Design review of the part built by this model. Coordinates are the model's own, in mm. Face numbers are marked on the shaded views. A direction names the side the tool comes from. Give positions to 0.01 mm unless a question says otherwise; leave off trailing zeros. Write each loop counter-clockwise with the first axis right and the second up, starting at its lowest first coordinate (ties: lowest second). Pieces come first, ordered by that corner, then holes. Notation, with made-up numbers: (50, 27.5) -> (105, 27.5) arc R14 ccw to (105, 33.5) -> close; hole circle Ø11 at (17, -11.5). An arc over 180 degrees is marked (long way). Return JSON: item names as keys, results as strings. Group by question number.
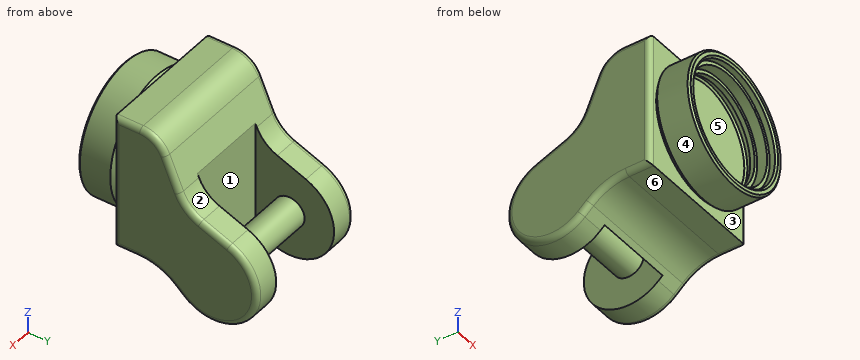
from build123d import *

# Parameters (mm, degrees)
CHAMFER1_SIZE           = 10
CHAMFER2_SIZE           = 5
CHAMFER3_SIZE           = 5
SKETCH4_R               = 160
BOSS_EXTRUDE1_DEPTH     = 5
BOSS_EXTRUDE2_DEPTH     = 187.5
FILLET1_R               = 15
SKETCH6_W               = 225
SKETCH6_H               = 220
CUT_EXTRUDE1_DEPTH      = 188.562818856
CUT_EXTRUDE1_DEPTH_BACK = 279.899051912
SKETCH7_R               = 42.5
BOSS_EXTRUDE3_DEPTH     = 225
SKETCH8_W               = 10
SKETCH8_H               = 12.5


with BuildPart() as part:
    # Sketch2 → Revolve1 (revolve)
    with BuildSketch(Plane.XY):
        Polygon((-160, 0), (-160, 20), (-150, 20), (-150, 80), (0, 80), (0, 100), (-180, 100), (-180, 0), align=None)
    revolve(axis=Axis((0, 100, 0), (0, -1, 0)))

    # Chamfer1
    chamfer1_edges = [part.edges().sort_by_distance(p)[0] for p in [
        (180, 100, 0),
    ]]
    chamfer(chamfer1_edges, length=CHAMFER1_SIZE)

    # Chamfer2
    chamfer2_edges = [part.edges().sort_by_distance(p)[0] for p in [
        (150, 80, 0),
        (160, 0, 0),
    ]]
    chamfer(chamfer2_edges, length=CHAMFER2_SIZE)

    # Chamfer3
    chamfer3_edges = [part.edges().sort_by_distance(p)[0] for p in [
        (180, 0, 0),
    ]]
    chamfer(chamfer3_edges, length=CHAMFER3_SIZE)

    # Sketch4 → Boss-Extrude1 (add)
    with BuildSketch(Plane(origin=(0, 100, 0), x_dir=(1, 0, 0), z_dir=(0, 1, 0))):
        Circle(SKETCH4_R)
    extrude(amount=BOSS_EXTRUDE1_DEPTH)

    # Sketch5 → Boss-Extrude2 (add, symmetric)
    with BuildSketch(Plane(origin=(0, 0, 0), x_dir=(0, 0, -1), z_dir=(1, 0, 0))):
        with BuildLine():
            Line((187.437181144, 105), (-187.562818856, 105))
            Line((-187.562818856, 105), (-187.562818856, 177.307219005))
            ThreePointArc((-187.562818856, 177.307219005), (-174.372707713, 221.312204528), (-139.151850084, 250.806423804))
            Line((-139.151850084, 250.806423804), (-49.751809858, 289.229433552))
            ThreePointArc((-49.751809858, 289.229433552), (-16.228261208, 312.275925599), (5.923948566, 346.397014559))
            Line((5.923948566, 346.397014559), (37.791857566, 426.304637395))
            ThreePointArc((37.791857566, 426.304637395), (219.726126853, 486.262863652), (247.066543683, 296.664422612))
            Line((247.066543683, 296.664422612), (225.636190899, 272.705721163))
            ThreePointArc((225.636190899, 272.705721163), (197.31197189, 226.228029294), (187.437181144, 172.703028297))
            Line((187.437181144, 172.703028297), (187.437181144, 105))
        make_face()
    extrude(amount=BOSS_EXTRUDE2_DEPTH, both=True)

    # Fillet1
    fillet1_edges = [part.edges().sort_by_distance(p)[0] for p in [
        (-187.5, 141.153609503, 187.562818856),
        (-187.5, 105, 0.062818856),
        (-187.5, 138.851514149, -187.437181144),
        (-187.5, 226.228029294, -197.31197189),
        (-187.5, 284.685071887, -236.351367291),
        (-187.5, 486.262863652, -219.726126853),
        (-187.5, 386.350825977, -21.857903066),
        (-187.5, 312.275925599, 16.228261208),
        (-187.5, 270.017928678, 94.451829971),
        (-187.5, 221.312204528, 174.372707713),
        (187.5, 141.153609503, 187.562818856),
        (187.5, 105, 0.062818856),
        (187.5, 138.851514149, -187.437181144),
        (187.5, 226.228029294, -197.31197189),
        (187.5, 284.685071887, -236.351367291),
        (187.5, 486.262863652, -219.726126853),
        (187.5, 386.350825977, -21.857903066),
        (187.5, 312.275925599, 16.228261208),
        (187.5, 270.017928678, 94.451829971),
        (187.5, 221.312204528, 174.372707713),
    ]]
    fillet(fillet1_edges, radius=FILLET1_R)

    # Sketch6 → Cut-Extrude1 (cut, two sides)
    with BuildSketch(Plane.XY) as cut_extrude1_sk:
        with Locations((0, 395)):
            Rectangle(SKETCH6_W, SKETCH6_H)
    extrude(amount=CUT_EXTRUDE1_DEPTH, mode=Mode.SUBTRACT)
    extrude(cut_extrude1_sk.sketch, amount=-CUT_EXTRUDE1_DEPTH_BACK, mode=Mode.SUBTRACT)

    # Sketch7 → Boss-Extrude3 (add)
    with BuildSketch(Plane.ZY.offset(-112.5)):
        with Locations((-153.899051812, 380)):
            Circle(SKETCH7_R)
    extrude(amount=BOSS_EXTRUDE3_DEPTH)

    # Sketch8 → Revolve2 (revolve)
    with BuildSketch(Plane.XY):
        with Locations((-145, 53.75)):
            Rectangle(SKETCH8_W, SKETCH8_H)
    revolve(axis=Axis((0, 0, 0), (0, 1, 0)))


solid = part.part
Q1. Insertion check: pin 1 (1 mm diameter, centred on x = -75, z = -202, fed in from -Y); pin 2 (1.5 mm diameter, centred on x = -83, z = 3, fed in from +Y); pin 3 (20.5 mm diameter, centred on x = -77, y = 151, fed in from -Z); pin 4 (8 mm diameter, centred on y = 162, z = -175, fed in from +X). Each pin has a flat end and moves straight along its axis. Give the tip position at first contact, or say it passes through.
Q2. Tool access review of the marked faces 1, 2 and 3: name each direction out of +Z, -Z, +X, -X, +Y, -Y from which nothing blocks a thin tool from reaching the whole face with its end or side.
Q3. Mouldability with a two-part tool opening along Z and no side actions: class the marked faces 4, 5 and 6 as +Z half, -Z half, draft (parallel to the pull), parting line (faces both ways), or undercut.
Q4. Take a section at A-A, the plane y = 40. Give the boundary of the cut face in (x, z), plus the area to 3 significant figures.
Q5. For L1, parallel to Z at x = 0, y = 55.75; L2, parallel to X at y = 64, z = 0; L3, parallel to Z at x = 0, y = 14.75, list the stretches that pass through material, from the lowest coordinate up. Write a range as from..to.
Final values:
{
 "1": {"pin 1": "stops at y = 236.12", "pin 2": "stops at y = 285", "pin 3": "stops at z = -187.44", "pin 4": "stops at x = 187.5"},
 "2": {"face 1": "+Z, -Z", "face 2": "+Z, +X, -X, +Y", "face 3": "none"},
 "3": {"face 4": "parting line", "face 5": "undercut", "face 6": "-Z half"},
 "4": {"outline": "circle Ø360 at (0, 0); hole circle Ø300 at (0, 0)", "area": "31,100 mm²"},
 "5": {"L1": "z = -180..-140, 140..180", "L2": "x = -180..-150, 150..180", "L3": "z = -180..-160, 160..180"}
}
